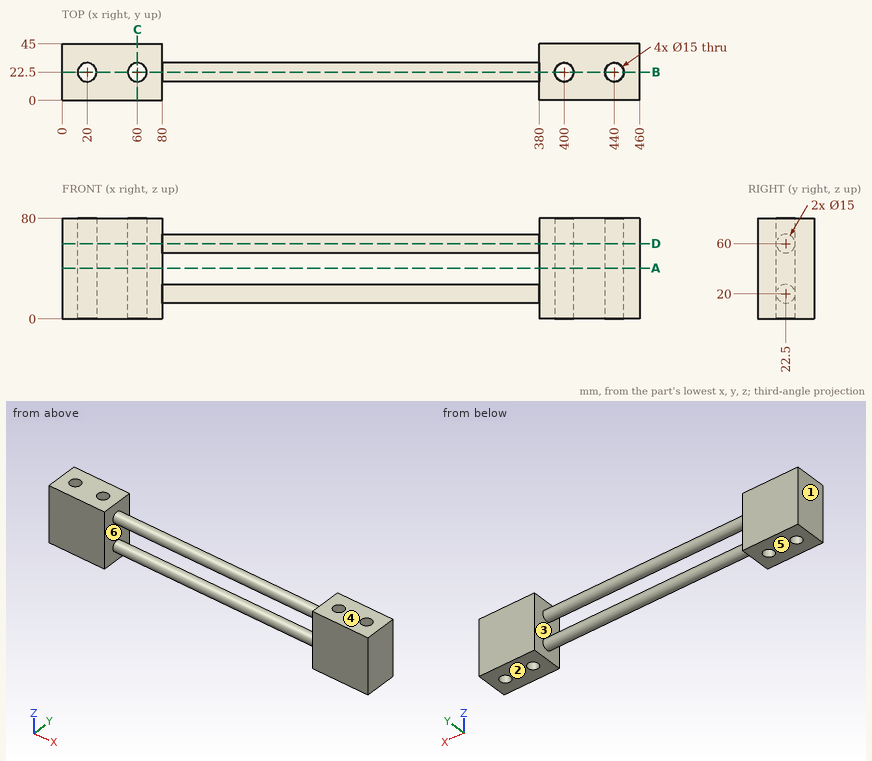
Can you work these out from the drawing? Everything is in mm from the part's minimum corner. A direction names the side the tool comes from. Give positions to 0.01 mm unless a question says otherwise; leave off trailing zeros. Loops run counter-clockwise (first coordinate to the right, second up) from the corner with the lowest first, then second, coordinate; pieces in that order, holes last. Notation, with made-up numbers: (-31, 11) -> (-7, 11) arc R19 ccw to (-7, 41) -> close; hole circle Ø11 at (16.5, -20.75). An arc over 180 degrees is marked (long way). Return JSON: item names as keys, results as strings.
Q1. I want a section at B-B, the plane y = 22.5. Count the separate pieces of the cut face and the enclosed holes in it, then the cut area to 3 significant figures.
Checks:
{"separate pieces": "5", "enclosed holes": "1", "area": "17,000 mm2"}
Q2. We'd pull the mould along Z, two halves only. Please class the marked faces 1, 2, 3 and 4: released by +Z, released by -Z, zero draft, split by the parting line, or undercut.
Checks:
{"face 1": "zero draft", "face 2": "released by -Z", "face 3": "undercut", "face 4": "released by +Z"}
Q3. For pin 1 Ø19.5 at (x, y) = (60, 22.5) entering from -Z; pin 2 Ø1.5 at (x, y) = (221.5, 15.5) entering from +Z; pin 3 Ø4 at (x, y) = (338.5, 22) entering from -Z; pin 4 Ø12 at (x, y) = (20, 22.5) entering from -Z, each with a flat end and sliding along its axis, tell me the tip position at first contact or that it passes through.
Checks:
{"pin 1": "stops at z = 0", "pin 2": "stops at z = 64.15", "pin 3": "stops at z = 12.5", "pin 4": "passes through"}
Q4. I want a section at A-A, the plane z = 40.5. List the corners of the cut face in (x, y) for me.
Checks:
{"outline": "(0, 0) -> (80, 0) -> (80, 45) -> (0, 45) -> close; (380, 0) -> (460, 0) -> (460, 45) -> (380, 45) -> close; hole circle Ø15 at (20, 22.5); hole circle Ø15 at (60, 22.5); hole circle Ø15 at (400, 22.5); hole circle Ø15 at (440, 22.5)"}
Q5. I want a section at D-D, the plane z = 60. List the corners of the cut face in (x, y) for me, then the cut area to 3 significant figures.
Checks:
{"outline": "(0, 0) -> (80, 0) -> (80, 15) -> (380, 15) -> (380, 0) -> (460, 0) -> (460, 45) -> (380, 45) -> (380, 30) -> (80, 30) -> (80, 45) -> (0, 45) -> close; hole circle Ø15 at (20, 22.5); hole circle Ø15 at (60, 22.5); hole circle Ø15 at (400, 22.5); hole circle Ø15 at (440, 22.5)", "area": "11,000 mm2"}
Q6. I want a section at C-C, the plane x = 60. List the corners of the cut face in (y, z) for me, then the cut area to 3 significant figures.
Checks:
{"outline": "(0, 0) -> (15, 0) -> (15, 80) -> (0, 80) -> close; (30, 0) -> (45, 0) -> (45, 80) -> (30, 80) -> close", "area": "2,400 mm2"}
Q7. I need wall thicknesses on probe 1 along X at (y, z) = (22, 71); probe 2 along Y at (x, z) = (440, 47); probe 3 along Z at (x, y) = (122.5, 22). Which ranges of each line are inside material? Lowest first, please.
Checks:
{"probe 1": "x = 0 to 12.52, 27.48 to 52.52, 67.48 to 80, 380 to 392.52, 407.48 to 432.52, 447.48 to 460", "probe 2": "y = 0 to 15, 30 to 45", "probe 3": "z = 12.52 to 27.48, 52.52 to 67.48"}
Q8. On a 3-axis mill with a long thin cutter (end or side, diameter ignored), from which of +Z, -Z, +X, -X, +Y, -Y can I reach the whole of each face in a straight line? I mean the marked faces 5 and 6. Say none if no direction works.
Checks:
{"face 5": "-Z, +X, -X, +Y, -Y", "face 6": "none"}
